Geometry: final body of the model. Coordinates: model frame, mm. Face numbers are marked on the shaded views. A direction names the side the tool comes from. Round coordinates to 2 decimals unless told otherwise and drop trailing zeros. Order: outer loops, then holes, each group sorted by start corner. A loop starts at its lowest first (then second) coordinate and runs counter-clockwise, first axis right, second up. Notation, with made-up numbers: M 13.25,5 L 26.25,5 A32 cw 26.25,36 Z; hole C 12,50 d6. An arc over 180 degrees is marked long. Return JSON: item names as keys, results as strings. Group by question number.
Q1. Access query for the marked faces 1, 2 and 3. Directions: +Z, -Z, +X, -X, +Y, -Y. A direction counts if a zero-diameter tool reaches every point of the face in a straight line with its end or side. Return the directions, or none.
Q2. Mould query, pull axis X, two halves, no side actions, for the marked faces 4, 5 and 6. Classes: released by +X, released by -X, zero draft, split by the parting line, or undercut.
Q3. Cut plane C-C on z = 4.75. Output: boundary loops of the cut face in (x, y).
Q4. Ray query, probe 1 along X at (y, z) = (0, 9.9); probe 2 along Y at (x, z) = (0, 4.25); probe 3 along X at (y, z) = (0, 7.5). Return the intervals inside material, ascending.
Q5. Contact query for flat-ended pins moving along their axis: pin 1 (15.5 mm diameter, centred on x = 9, y = -5, fed in from +Z); pin 2 (5 mm diameter, centred on x = 19.5, z = 3.5, fed in from -Y); pin 3 (18 mm diameter, centred on x = 0, y = 0, fed in from -Z); pin 4 (4 mm diameter, centred on x = 3, z = 7.5, fed in from +Y). Output: stop coordinate, or through.
Q6. Cut plane A-A on x = 0. Output: boundary loops of the cut face in (y, z), and give its area (3 significant figures).
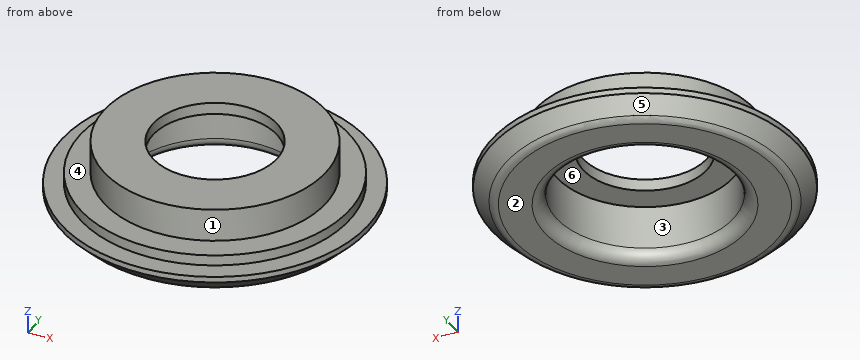
```python
from build123d import *


with BuildPart() as f1:
    # F0 (on Front) → F1 (revolve)
    with BuildSketch(Plane.XZ):
        with BuildLine():
            Line((-22.071573, 0), (-17, 0))
            ThreePointArc((-17, 0), (-15.585786, 0.585786), (-15, 2))
            Line((-15, 2), (-15, 9.4))
            Line((-15, 9.4), (-10.5, 9.4))
            Line((-10.5, 9.4), (-10.5, 11.4))
            Line((-10.5, 11.4), (-18.75, 11.4))
            Line((-18.75, 11.4), (-18.75, 5.8))
            Line((-18.75, 5.8), (-22.75, 5.8))
            Line((-22.75, 5.8), (-22.75, 4))
            Line((-22.75, 4), (-25.9, 4))
            Line((-25.9, 4), (-25.9, 3))
            Line((-25.9, 3), (-23.485786, 0.585786))
            ThreePointArc((-23.485786, 0.585786), (-22.83694, 0.152241), (-22.071573, 0))
        make_face()
    revolve(axis=Axis((0, 0, 5.7), (0, 0, 1)))


solid = f1.part
```
Result sheet:
{
 "1": {"face 1": "+Z", "face 2": "-Z, +X, -X, +Y, -Y", "face 3": "-Z"},
 "2": {"face 4": "zero draft", "face 5": "split by the parting line", "face 6": "undercut"},
 "3": {"outline": "C 0,0 d45.5; hole C 0,0 d30"},
 "4": {"probe 1": "x = -18.75 to -10.5, 10.5 to 18.75", "probe 2": "y = -22.75 to -15, 15 to 22.75", "probe 3": "x = -18.75 to -15, 15 to 18.75"},
 "5": {"pin 1": "stops at z = 11.4", "pin 2": "stops at y = -19.54", "pin 3": "passes through", "pin 4": "stops at y = 22.67"},
 "6": {"outline": "M -25.9,3 L -23.49,0.59 A2 ccw -22.07,0 L -17,0 A2 ccw -15,2 L -15,9.4 L -10.5,9.4 L -10.5,11.4 L -18.75,11.4 L -18.75,5.8 L -22.75,5.8 L -22.75,4 L -25.9,4 Z; M 10.5,9.4 L 15,9.4 L 15,2 A2 ccw 17,0 L 22.07,0 A2 ccw 23.49,0.59 L 25.9,3 L 25.9,4 L 22.75,4 L 22.75,5.8 L 18.75,5.8 L 18.75,11.4 L 10.5,11.4 Z", "area": "164 mm²"}
}
